Verification items for this drawing (mm, ordinates from the low corner). Coordinates: 2 decimals unless noted, no trailing zeros. Loops run counter-clockwise (first coordinate to the right, second up) from the corner with the lowest first, then second, coordinate; pieces in that order, holes last. Notation, with made-up numbers: (38.25, 2.25) - (79.25, 2.25) arc R15 cw to (79.25, 20.25) - close; hole circle Ø4 at (-37, 45.5). An arc over 180 degrees is marked (long way). One line per item, written item: value. Start each with the question number.
(1) Section check B-B (x = 16). Record the boundary of the cut face in (y, z).
(2) Thickness scan on probe 1 along Z at (x, y) = (10.5, 14). Record the ranges inside material, lowest first. Write a range as [from, to].
(3) Gauge pin test, flat ends, axial feed: P1, Ø6, axis at x = 21.5, y = 15, coming from the -Z side; P2, Ø8, axis at x = 13, z = 20.5, coming from the -Y side. Record the tip position at first contact, or that the pin passes through.
(4) Section check A-A (y = 13). Record the boundary of the cut face in (x, z).
(5) Section check C-C (z = 9.5). Record the boundary of the cut face in (x, y), plus the area to 3 significant figures.
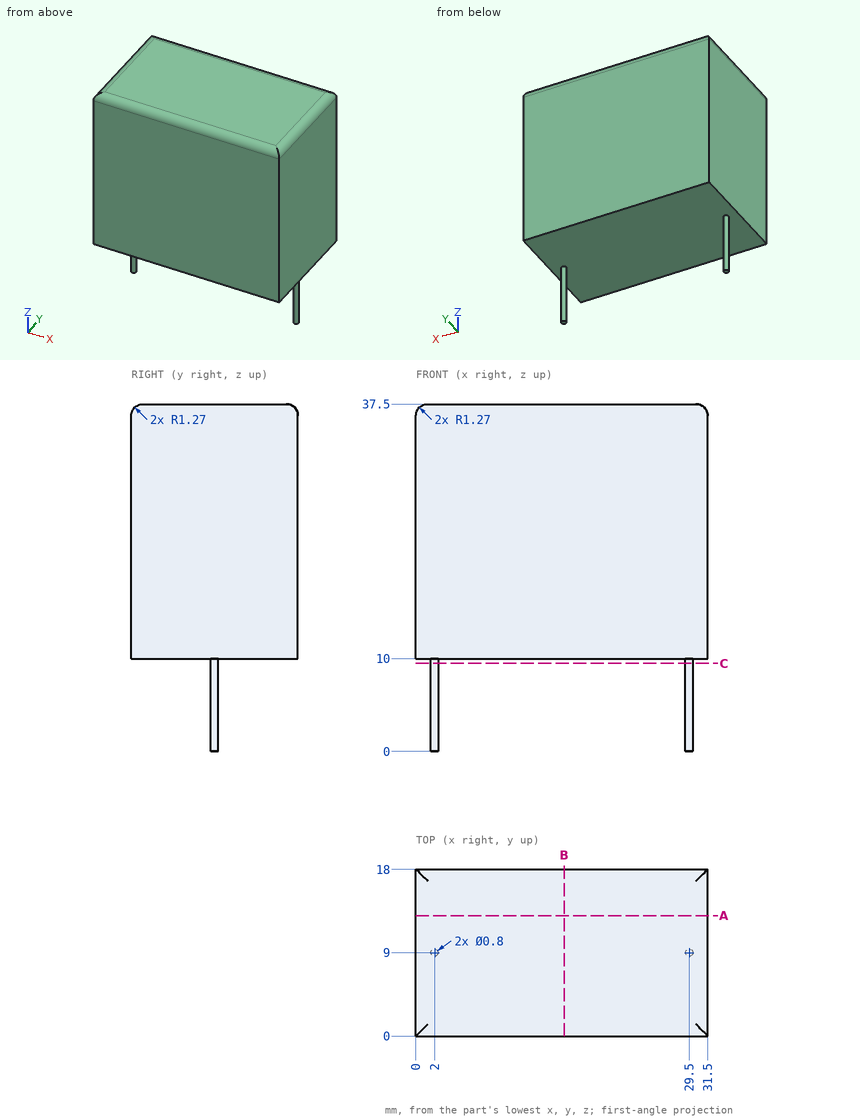
Responses:
1. outline: (0, 10) - (18, 10) - (18, 36.23) arc R1.27 ccw to (16.73, 37.5) - (1.27, 37.5) arc R1.27 ccw to (0, 36.23) - close
2. probe 1: z = [10, 37.5]
3. P1: stops at z = 10
3. P2: stops at y = 0
4. outline: (0, 10) - (31.5, 10) - (31.5, 36.23) arc R1.27 ccw to (30.23, 37.5) - (1.27, 37.5) arc R1.27 ccw to (0, 36.23) - close
5. outline: circle Ø0.8 at (2, 9); circle Ø0.8 at (29.5, 9)
5. area: 1.01 mm²
